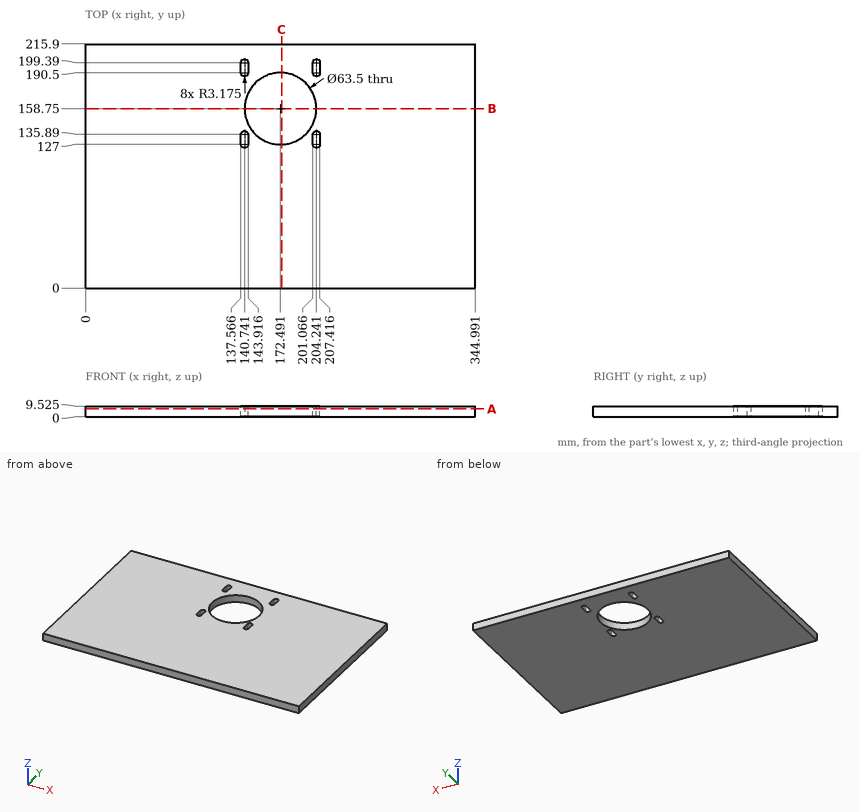
Study the drawing (mm; zero at the part's minimum x, y, z) and answer. Round coordinates to 2 decimals unless told otherwise and drop trailing zeros. Write each loop counter-clockwise with the first axis right and the second up, starting at its lowest first coordinate (ties: lowest second). Pieces come first, ordered by that corner, then holes. Notation, with made-up numbers: (-13, 67.25) -> (12, 67.25) arc R28 ccw to (12, 87.25) -> close; hole circle Ø4 at (43.5, 35). An arc over 180 degrees is marked (long way). Answer as CSV lines item,"result". Start each with the question number.
(1) The part is cut by section C-C, the plane x = 173.5. Give the vertices of the cut face in (y, z) (1 decimal).
(2) The part is cut by section A-A, the plane z = 7. Give the number of separate pieces and of enclosed holes in the cut face, then the cut area to 3 significant figures.
(3) The part is cut by section B-B, the plane y = 158.75. Give the vertices of the cut face in (x, z) (1 decimal).
(4) Find the intervals of material crossed by probe 1 along X at (y, z) = (181, 3); probe 2 along Y at (x, z) = (196, 2.25); probe 3 along Y at (x, z) = (144, 4.5), in increasing order.
Output values:
1,outline,"(0, 0) -> (127, 0) -> (127, 9.5) -> (0, 9.5) -> close; (190.5, 0) -> (215.9, 0) -> (215.9, 9.5) -> (190.5, 9.5) -> close"
2,separate pieces,"1"
2,enclosed holes,"5"
2,area,"71,000 mm²"
3,outline,"(0, 0) -> (140.7, 0) -> (140.7, 9.5) -> (0, 9.5) -> close; (204.2, 0) -> (345, 0) -> (345, 9.5) -> (204.2, 9.5) -> close"
4,probe 1,"x = 0 to 149.84, 195.14 to 344.99"
4,probe 2,"y = 0 to 137.41, 180.09 to 215.9"
4,probe 3,"y = 0 to 144.74, 172.76 to 215.9"
